Here's how the part is built. I have some questions about the finished solid (model axes, mm). A direction names the side the tool comes from. Round coordinates to 2 decimals unless told otherwise and drop trailing zeros. Write each loop counter-clockwise with the first axis right and the second up, starting at its lowest first coordinate (ties: lowest second). Pieces come first, ordered by that corner, then holes. Notation, with made-up numbers: (68, -16) -> (93, -16) arc R5 cw to (93, -7) -> close; hole circle Ø8 at (79, -31.5). An arc over 180 degrees is marked (long way). Put each result on its own line as item: value. Start each with the question number.
1. We'd pull the mould along Z, two halves only. Please class faces 4 (the face through (-97.719, -54.494, 1.191)), 5 (the face through (1.288, -55.096, 6.639)), 6 (the face through (95.057, 35.034, 2.948)): +Z half, -Z half, draft (parallel to the pull), parting line (faces both ways), or undercut.
2. For pin 1 (2 mm diameter, centred on y = -34, z = 7.5, fed in from +X); pin 2 (3 mm diameter, centred on y = 34.6, z = 4.9, fed in from +X); pin 3 (4 mm diameter, centred on x = -95.5, z = 4.5, fed in from +Y), each with a flat end and sliding along its axis, tell me the tip position at first contact or that it passes through.
3. Which directions (+Z, -Z, +X, -X, +Y, -Y) give clear straight access to the entire face, cutting with the end or side of a thin tool? Please do faces 1 (the face through (90, 35, 5)), 2 (the face through (81.556, 44.043, 8.104)), 3 (the face through (-99, -4.6, 7)).
4. Suppose I cut it at B-B (y = 34.6). Please give me the cut outline in (x, z).
5. Suppose I cut it at A-A (x = 87.4). Please give me the cut outline in (y, z), then the cut area to 3 significant figures.
6. I need wall thicknesses on probe 1 along Z at (x, y) = (92.5, 34.6); probe 2 along Y at (x, z) = (78.5, 3); probe 3 along Z at (x, y) = (95, 34). Which ranges of each line are inside material? Lowest first, please. Write a range as from..to.
```python
from build123d import *

# Parameters (mm, degrees)
F0_W      = 200
F0_H      = 113.8
F1_DEPTH  = 8.35
F2_R      = 8
F3_R      = 6
F5_R      = 5.85
F6_DEPTH  = 0.5
F8_R      = 2
F9_DEPTH  = 10
F12_W     = 9.2
F12_H     = 5.3
F13_DEPTH = 25


with BuildPart() as f1:
    # F0 (on Top) → F1 (new body)
    with BuildSketch(Plane.XY):
        Rectangle(F0_W, F0_H)
    extrude(amount=F1_DEPTH)

    # F2
    f2_edges = [f1.edges().sort_by_distance(p)[0] for p in [
        (-100, -56.9, 4.175),
        (100, -56.9, 4.175),
        (-100, 56.9, 4.175),
        (100, 56.9, 4.175),
    ]]
    fillet(f2_edges, radius=F2_R)

    # F3
    f3_edges = [f1.edges().sort_by_distance(p)[0] for p in [
        (100, 0, 8.35),
        (97.656854, -54.556854, 8.35),
        (97.656854, 54.556854, 8.35),
        (0, -56.9, 8.35),
        (0, 56.9, 8.35),
        (-97.656854, -54.556854, 8.35),
        (-97.656854, 54.556854, 8.35),
    ]]
    fillet(f3_edges, radius=F3_R)

    # F5 (on face) → F6 (cut)
    with BuildSketch(Plane(origin=(0, 0, 8.35), x_dir=(1, 0, 0), z_dir=(0, 0, -1))):
        with Locations((87.4, -44.3)):
            Circle(F5_R)
    extrude(amount=F6_DEPTH, mode=Mode.SUBTRACT)

    # F8 (on face) → F9 (cut)
    with BuildSketch(Plane(origin=(100, 0, 0), x_dir=(0, -1, 0), z_dir=(-1, 0, 0))):
        with Locations((-34.6, 4.9)):
            Circle(F8_R)
    extrude(amount=F9_DEPTH, mode=Mode.SUBTRACT)

    # F12 (on face) → F13 (join)
    with BuildSketch(Plane.YZ.offset(-100)):
        with Locations((0, 5.7)):
            Rectangle(F12_W, F12_H)
    extrude(amount=F13_DEPTH)


solid = f1.part
```
Verdict:
1. face 4: draft
1. face 5: +Z half
1. face 6: undercut
2. pin 1: stops at x = 98.33
2. pin 2: stops at x = 90
2. pin 3: stops at y = 56.59
3. face 1: +X
3. face 2: +Z
3. face 3: +Z, -X, -Y
4. outline: (-100, 0) -> (100, 0) -> (100, 2.35) arc R6 ccw to (99.97, 2.9) -> (90, 2.9) -> (90, 6.9) -> (97.91, 6.9) arc R6 ccw to (94, 8.35) -> (-94, 8.35) arc R6 ccw to (-100, 2.35) -> close
5. outline: (-56.9, 0) -> (56.9, 0) -> (56.9, 2.35) arc R6 ccw to (50.9, 8.35) -> (50.15, 8.35) -> (50.15, 7.85) -> (38.45, 7.85) -> (38.45, 8.35) -> (-50.9, 8.35) arc R6 ccw to (-56.9, 2.35) -> close
5. area: 929 mm^2
6. probe 1: z = 0..2.9, 6.9..8.35
6. probe 2: y = -56.86..56.86
6. probe 3: z = 0..2.99, 6.81..8.27
